Geometry check sheet. Reference: drawing and pictorial views, mm from the part's lowest x, y, z. A direction names the side the tool comes from. Coordinates: 2 decimals unless noted, no trailing zeros. Loops run counter-clockwise (first coordinate to the right, second up) from the corner with the lowest first, then second, coordinate; pieces in that order, holes last. Notation, with made-up numbers: (-18.5, 51) - (14.5, 51) arc R23 cw to (14.5, 75) - close; hole circle Ø9 at (26, -27). An arc over 180 degrees is marked (long way). Use a Markdown table: item, result. Add a question column.
1) Go/stop test with flat-tipped pins: P1, Ø4, axis at x = 13.5, z = 45.5, coming from the -Y side; P2, Ø10, axis at x = 39.5, z = 50, coming from the +Y side; P3, Ø2, axis at x = 19, y = 35, coming from the -Z side. Record where each tip stops, or that it passes through.
2) Sectioned sample at A-A, the plane x = 25. Enter the section's corners in (y, z).
3) Tool access check on the marked faces 4 and 5. Record the directions out of +Z, -Z, +X, -X, +Y, -Y that give a thin tool (end or side, any length) a straight path to the whole face; none if there is none.
4) Thickness scan on line 1 (Y direction, x = 25, z = 32); line 2 (Y direction, x = 25, z = 58.15); line 3 (Z direction, x = 19, y = 44.5). Record the ranges inside material, lowest first.
5) Sectioned sample at B-B, the plane y = 35. Enter the section's corners in (x, z).
6) Draft check along X on the marked faces 1, 2 and 3. Enter one of: pulls with the +X half, pulls with the -X half, needs draft (parallel to the pull), parting line crosses it, or undercut.
7) Sectioned sample at C-C, the plane y = 23. Enter the section's corners in (x, z).
8) Sectioned sample at D-D, the plane z = 52. Enter the section's corners in (x, y), then the cut area to 3 significant figures.
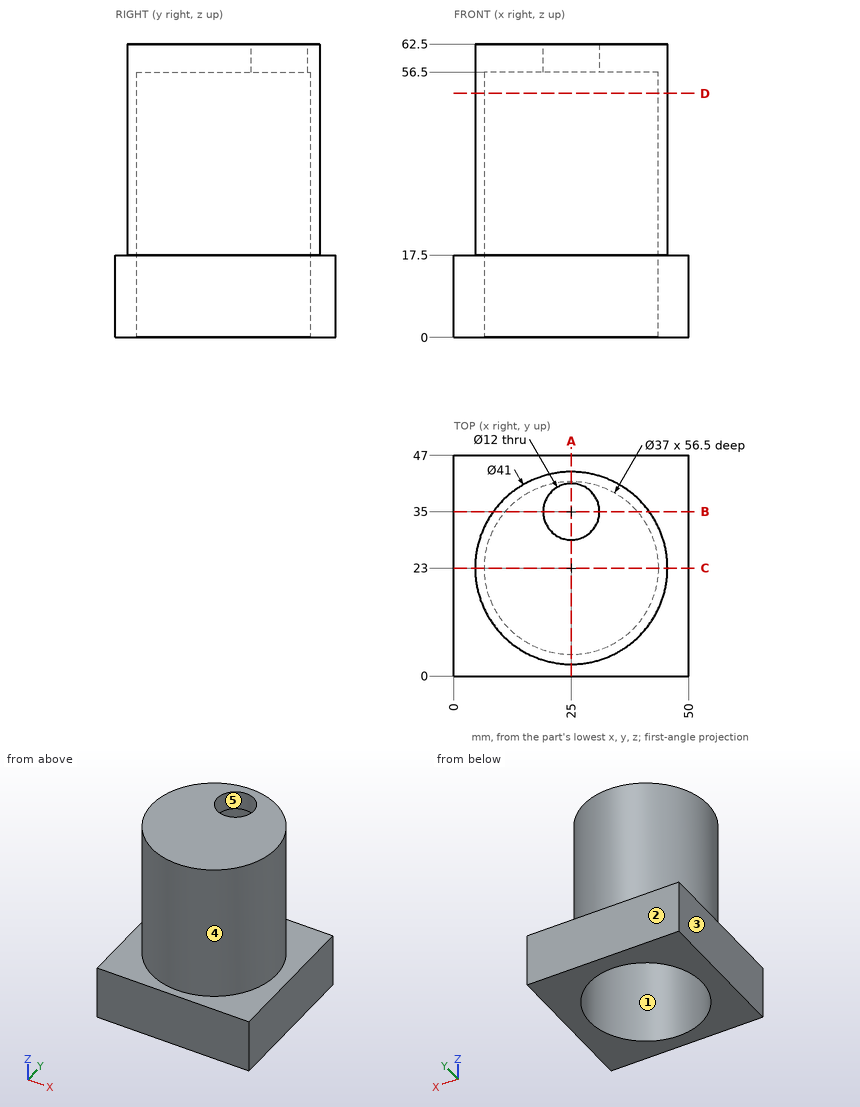
Solved:
| question | item | result |
|---|---|---|
| 1 | P1 | stops at y = 4.83 |
| 1 | P2 | stops at y = 41.17 |
| 1 | P3 | stops at z = 56.5 |
| 2 | outline | (0, 0) - (4.5, 0) - (4.5, 56.5) - (29, 56.5) - (29, 62.5) - (2.5, 62.5) - (2.5, 17.5) - (0, 17.5) - close; (41, 56.5) - (41.5, 56.5) - (41.5, 0) - (47, 0) - (47, 17.5) - (43.5, 17.5) - (43.5, 62.5) - (41, 62.5) - close |
| 3 | face 4 | +Z |
| 3 | face 5 | +Z, -Z |
| 4 | line 1 | y = 2.5 to 4.5, 41.5 to 43.5 |
| 4 | line 2 | y = 2.5 to 29, 41 to 43.5 |
| 4 | line 3 | z = 0 to 17.5 |
| 5 | outline | (0, 0) - (10.92, 0) - (10.92, 56.5) - (19, 56.5) - (19, 62.5) - (8.38, 62.5) - (8.38, 17.5) - (0, 17.5) - close; (31, 56.5) - (39.08, 56.5) - (39.08, 0) - (50, 0) - (50, 17.5) - (41.62, 17.5) - (41.62, 62.5) - (31, 62.5) - close |
| 6 | face 1 | undercut |
| 6 | face 2 | needs draft |
| 6 | face 3 | pulls with the -X half |
| 7 | outline | (0, 0) - (6.5, 0) - (6.5, 56.5) - (43.5, 56.5) - (43.5, 0) - (50, 0) - (50, 17.5) - (45.5, 17.5) - (45.5, 62.5) - (4.5, 62.5) - (4.5, 17.5) - (0, 17.5) - close |
| 8 | outline | circle Ø41 at (25, 23); hole circle Ø37 at (25, 23) |
| 8 | area | 245 mm2 |
